from build123d import *

# Parameters (mm, degrees)
SKETCH1_R                   = 4.8
BOSS_EXTRUDE1_DEPTH         = 4
SKETCH3_R                   = 1.5
BOSS_EXTRUDE2_DEPTH         = 2
BOSS_EXTRUDE3_DEPTH         = 1.1
M1_4X0_3_TAPPED_HOLE2_D     = 1.1
M1_4X0_3_TAPPED_HOLE2_DEPTH = 1.1
SKETCH14_R                  = 0.5
BOSS_EXTRUDE4_DEPTH         = 4.5
SKETCH15_R                  = 1.75
BOSS_EXTRUDE5_DEPTH         = 1.4


with BuildPart() as part:
    # Sketch1 → Boss-Extrude1 (new body)
    with BuildSketch(Plane.XY):
        Circle(SKETCH1_R)
    extrude(amount=BOSS_EXTRUDE1_DEPTH)

    # Sketch3 → Boss-Extrude2 (add)
    with BuildSketch(Plane.XY.offset(4)):
        Circle(SKETCH3_R)
    extrude(amount=BOSS_EXTRUDE2_DEPTH)

    # Sketch4 → Boss-Extrude3 (add)
    with BuildSketch(Plane.XY.offset(6)):
        with BuildLine():
            Line((0, 3.3), (0, 2.5))
            ThreePointArc((0, 2.5), (1.250000026, 2.165063495), (2.165063539, 1.249999948))
            ThreePointArc((2.165063539, 1.249999948), (1.724566258, 2.23997367), (1.5, 3.3))
            Line((1.5, 3.3), (0, 3.3))
        make_face()
        with BuildLine():
            Line((0, 4.3), (0, 3.3))
            Line((0, 3.3), (1.5, 3.3))
            ThreePointArc((1.5, 3.3), (0.901387819, 4.027081728), (0, 4.3))
        make_face()
        with BuildLine():
            Line((-1.5, 3.3), (0, 3.3))
            Line((0, 3.3), (0, 4.3))
            ThreePointArc((0, 4.3), (-0.901387819, 4.027081728), (-1.5, 3.3))
        make_face()
        with BuildLine():
            ThreePointArc((-2.165063492, 1.25000003), (-1.249999985, 2.165063518), (0, 2.5))
            Line((0, 2.5), (0, 3.3))
            Line((0, 3.3), (-1.5, 3.3))
            ThreePointArc((-1.5, 3.3), (-1.724566244, 2.239973715), (-2.165063492, 1.25000003))
        make_face()
        with BuildLine():
            ThreePointArc((-1.299038106, 0.75), (-0.75, 1.299038106), (0, 1.5))
            Line((0, 1.5), (0, 2.5))
            ThreePointArc((0, 2.5), (-1.249999985, 2.165063518), (-2.165063492, 1.25000003))
            ThreePointArc((-2.165063492, 1.25000003), (-2.5, 1.7e-08), (-2.165063509, -1.25))
            Line((-2.165063509, -1.25), (-1.299038106, -0.75))
            ThreePointArc((-1.299038106, -0.75), (-1.5, 0), (-1.299038106, 0.75))
        make_face()
        with BuildLine():
            Line((0, 2.5), (0, 1.5))
            ThreePointArc((0, 1.5), (0.75, 1.299038106), (1.299038106, 0.75))
            ThreePointArc((1.299038106, 0.75), (1.448888739, 0.388228568), (1.5, 0))
            ThreePointArc((1.5, 0), (1.448888739, -0.388228568), (1.299038106, -0.75))
            Line((1.299038106, -0.75), (2.165063509, -1.25))
            ThreePointArc((2.165063509, -1.25), (2.414814566, -0.647047613), (2.5, 0))
            ThreePointArc((2.5, 0), (2.414814573, 0.647047584), (2.165063539, 1.249999948))
            ThreePointArc((2.165063539, 1.249999948), (1.250000026, 2.165063495), (0, 2.5))
        make_face()
        with BuildLine():
            Line((1.299038106, 0.75), (0, 0))
            Line((0, 0), (1.299038106, -0.75))
            ThreePointArc((1.299038106, -0.75), (1.448888739, -0.388228568), (1.5, 0))
            ThreePointArc((1.5, 0), (1.448888739, 0.388228568), (1.299038106, 0.75))
        make_face()
        with BuildLine():
            Line((0, 1.5), (0, 0))
            Line((0, 0), (1.299038106, 0.75))
            ThreePointArc((1.299038106, 0.75), (0.75, 1.299038106), (0, 1.5))
        make_face()
        with BuildLine():
            Line((-1.299038106, 0.75), (0, 0))
            Line((0, 0), (0, 1.5))
            ThreePointArc((0, 1.5), (-0.75, 1.299038106), (-1.299038106, 0.75))
        make_face()
        with BuildLine():
            Line((-1.299038106, -0.75), (0, 0))
            Line((0, 0), (-1.299038106, 0.75))
            ThreePointArc((-1.299038106, 0.75), (-1.5, 0), (-1.299038106, -0.75))
        make_face()
        with BuildLine():
            Line((0, -1.5), (0, 0))
            Line((0, 0), (-1.299038106, -0.75))
            ThreePointArc((-1.299038106, -0.75), (-0.75, -1.299038106), (0, -1.5))
        make_face()
        with BuildLine():
            Line((1.299038106, -0.75), (0, 0))
            Line((0, 0), (0, -1.5))
            ThreePointArc((0, -1.5), (0.75, -1.299038106), (1.299038106, -0.75))
        make_face()
        with BuildLine():
            ThreePointArc((0, -1.5), (-0.75, -1.299038106), (-1.299038106, -0.75))
            Line((-1.299038106, -0.75), (-2.165063509, -1.25))
            ThreePointArc((-2.165063509, -1.25), (-1.25, -2.165063509), (0, -2.5))
            ThreePointArc((0, -2.5), (1.25, -2.165063509), (2.165063509, -1.25))
            Line((2.165063509, -1.25), (1.299038106, -0.75))
            ThreePointArc((1.299038106, -0.75), (0.75, -1.299038106), (0, -1.5))
        make_face()
        with BuildLine():
            ThreePointArc((2.5, 0), (2.414814566, -0.647047613), (2.165063509, -1.25))
            Line((2.165063509, -1.25), (2.857883832, -1.65))
            Line((2.857883832, -1.65), (3.607883832, -0.350961894))
            ThreePointArc((3.607883832, -0.350961894), (2.802157271, 0.373531311), (2.165063539, 1.249999948))
            ThreePointArc((2.165063539, 1.249999948), (2.414814573, 0.647047584), (2.5, 0))
        make_face()
        with BuildLine():
            Line((2.857883832, -1.65), (2.165063509, -1.25))
            ThreePointArc((2.165063509, -1.25), (1.25, -2.165063509), (0, -2.5))
            ThreePointArc((0, -2.5), (1.077591002, -2.613505032), (2.107883832, -2.949038106))
            Line((2.107883832, -2.949038106), (2.857883832, -1.65))
        make_face()
        with BuildLine():
            ThreePointArc((0, -2.5), (-1.25, -2.165063509), (-2.165063509, -1.25))
            Line((-2.165063509, -1.25), (-2.857883832, -1.65))
            Line((-2.857883832, -1.65), (-2.107883832, -2.949038106))
            ThreePointArc((-2.107883832, -2.949038106), (-1.077591002, -2.613505032), (0, -2.5))
        make_face()
        with BuildLine():
            Line((-2.857883832, -1.65), (-2.165063509, -1.25))
            ThreePointArc((-2.165063509, -1.25), (-2.5, 1.7e-08), (-2.165063492, 1.25000003))
            ThreePointArc((-2.165063492, 1.25000003), (-2.80215724, 0.373531346), (-3.607883832, -0.350961894))
            Line((-3.607883832, -0.350961894), (-2.857883832, -1.65))
        make_face()
        with BuildLine():
            Line((-3.723909236, -2.15), (-2.857883832, -1.65))
            Line((-2.857883832, -1.65), (-3.607883832, -0.350961894))
            ThreePointArc((-3.607883832, -0.350961894), (-3.938248989, -1.232916114), (-3.723909236, -2.15))
        make_face()
        with BuildLine():
            Line((-2.107883832, -2.949038106), (-2.857883832, -1.65))
            Line((-2.857883832, -1.65), (-3.723909236, -2.15))
            ThreePointArc((-3.723909236, -2.15), (-3.03686117, -2.794165614), (-2.107883832, -2.949038106))
        make_face()
        with BuildLine():
            Line((3.723909236, -2.15), (2.857883832, -1.65))
            Line((2.857883832, -1.65), (2.107883832, -2.949038106))
            ThreePointArc((2.107883832, -2.949038106), (3.03686117, -2.794165614), (3.723909236, -2.15))
        make_face()
        with BuildLine():
            Line((3.607883832, -0.350961894), (2.857883832, -1.65))
            Line((2.857883832, -1.65), (3.723909236, -2.15))
            ThreePointArc((3.723909236, -2.15), (3.938248989, -1.232916114), (3.607883832, -0.350961894))
        make_face()
    extrude(amount=BOSS_EXTRUDE3_DEPTH)

    # M1.4x0.3 Tapped Hole2
    with Locations(Plane.XY.offset(7.1)):
        with Locations((2.857884156, -1.649999841), (-2.85788391, -1.649999841), (0, 3.300000228)):
            Hole(M1_4X0_3_TAPPED_HOLE2_D / 2, depth=M1_4X0_3_TAPPED_HOLE2_DEPTH)

    # Sketch14 → Boss-Extrude4 (add)
    with BuildSketch(Plane(origin=(0, 0, 0), x_dir=(-1, 0, 0), z_dir=(0, 0, -1))):
        Circle(SKETCH14_R)
    extrude(amount=BOSS_EXTRUDE4_DEPTH)

    # Sketch15 → Boss-Extrude5 (add)
    with BuildSketch(Plane.XY.offset(7.1)):
        Circle(SKETCH15_R)
    extrude(amount=BOSS_EXTRUDE5_DEPTH)


solid = part.part
Verification items for the finished model (mm, model axes). A direction names the side the tool comes from. Round coordinates to 2 decimals unless told otherwise and drop trailing zeros. Order: outer loops, then holes, each group sorted by start corner. A loop starts at its lowest first (then second) coordinate and runs counter-clockwise, first axis right, second up. Notation, with made-up numbers: (66, 61.5) -> (109, 61.5) arc R28 cw to (109, 90.5) -> close; hole circle Ø11 at (5, 45). An arc over 180 degrees is marked (long way). Put each result on its own line as item: value.
1) Section check A-A (x = -3). Record the cut outline in (y, z).
Final values:
outline: (-3.75, 0) -> (3.75, 0) -> (3.75, 4) -> (-3.75, 4) -> close; (-2.81, 6) -> (-2.18, 6) -> (-2.18, 7.1) -> (-2.81, 7.1) -> close; (-1.12, 6) -> (0.17, 6) -> (0.17, 7.1) -> (-1.12, 7.1) -> close
2) Mould release check, pull along X, two halves, no side actions. Record for faces 5 (the flat face through (0, 0, -4.5)), 6 (the cylindrical face through (2.58, 4.05, 1.97)), 7 (the cylindrical face through (2.35, -1.86, 6.54)): +X half, -X half, draft (parallel to the pull), parting line (faces both ways), or undercut.
Final values:
face 5: draft
face 6: parting line
face 7: undercut
3) Section check B-B (z = 4.25). Record the cut outline in (x, y), then the cut area to 3 significant figures.
Final values:
outline: circle Ø3 at (0, 0)
area: 7.07 mm^2
4) Section check C-C (x = 1). Record the cut outline in (y, z).
Final values:
outline: (-4.69, 0) -> (4.69, 0) -> (4.69, 4) -> (1.12, 4) -> (1.12, 6) -> (3.96, 6) -> (3.96, 7.1) -> (1.44, 7.1) -> (1.44, 8.5) -> (-1.44, 8.5) -> (-1.44, 7.1) -> (-2.6, 7.1) -> (-2.6, 6) -> (-1.12, 6) -> (-1.12, 4) -> (-4.69, 4) -> close
5) Section check D-D (y = -3.25). Record the cut outline in (x, z).
Final values:
outline: (-3.53, 0) -> (3.53, 0) -> (3.53, 4) -> (-3.53, 4) -> close
6) Material ranges on line 1 (Z direction, x = 2, y = -0.25); line 2 (Z direction, x = -3, y = 1.5); line 3 (X direction, y = 0.75, z = 2.5), recorded low to high.
Final values:
line 1: z = 0 to 4, 6 to 7.1
line 2: z = 0 to 4
line 3: x = -4.74 to 4.74
7) Set-up check for faces 1 (the cylindrical face through (0.119, 2.763, 6.542)), 2 (the cylindrical face through (0.108, -0.488, -2.218)), 3 (the flat face through (0, 2, 6)), 4 (the flat face through (0, 0, 8.5)): record each of +Z, -Z, +X, -X, +Y, -Y from which the full face is reachable in a straight line by a thin tool's end or side.
Final values:
face 1: +Z
face 2: -Z
face 3: none
face 4: +Z, +X, -X, +Y, -Y
8) Depth check by flat-ended pin: pin 1 (3 mm diameter, centred on x = 0.5, y = 2.5, fed in from +Z); pin 2 (2 mm diameter, centred on y = 2, z = -3, fed in from -X); pin 3 (1.3 mm diameter, centred on x = -2.86, y = -1.65, fed in from -Z); pin 4 (1.5 mm diameter, centred on y = -3.5, z = 6, fed in from +X). Enter the tip coordinate at first touch or a pass-through.
Final values:
pin 1: stops at z = 8.5
pin 2: passes through
pin 3: stops at z = 0
pin 4: stops at x = 3.12
